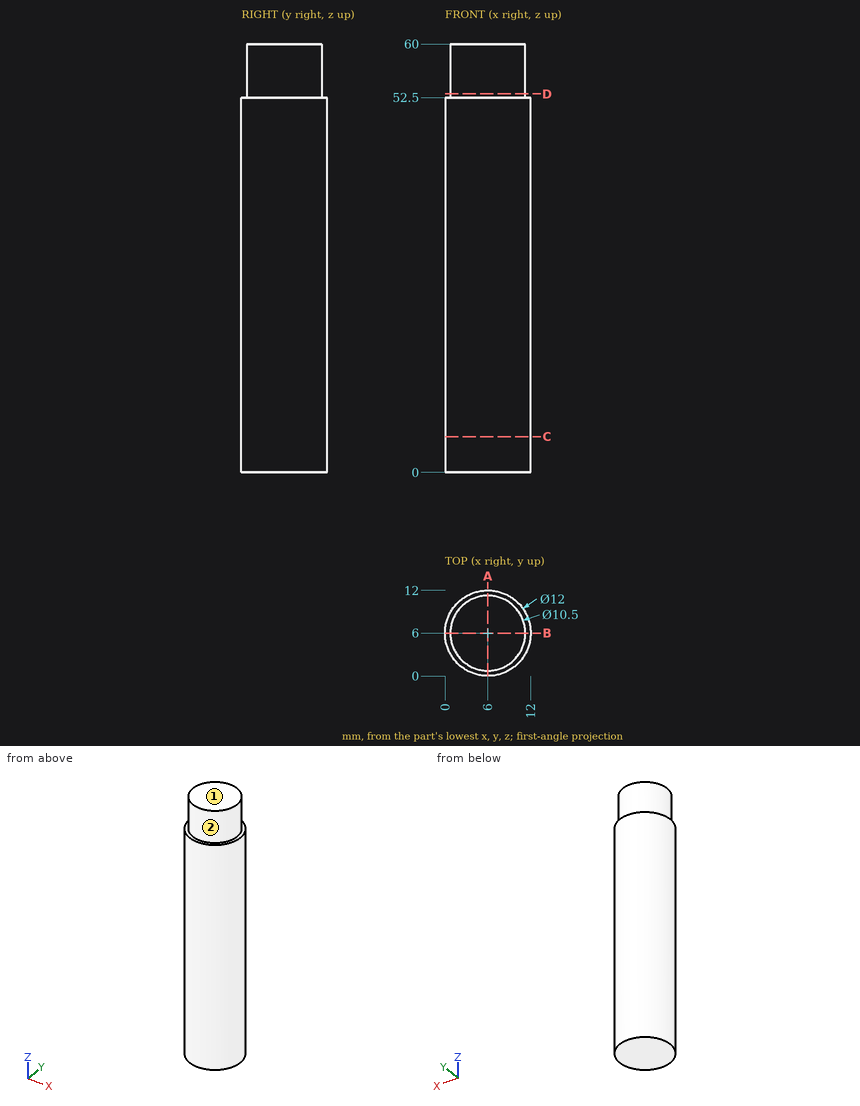
Here's the drawing with two shaded views (mm, measured from the low corner). I have some questions. A direction names the side the tool comes from. Give positions to 0.01 mm unless a question says otherwise; leave off trailing zeros. Loops run counter-clockwise (first coordinate to the right, second up) from the corner with the lowest first, then second, coordinate; pieces in that order, holes last. Notation, with made-up numbers: M 21,-31 L 72,-31 A35 cw 72,7 Z; hole C 78.25,89 d3. An arc over 180 degrees is marked long. Use one line per item in the form item = value. Start each with the question number.
(1) Please list where these lines run through material, in increasing order: line 1 (Z direction, x = 6.25, y = 11.5); line 2 (X direction, y = 5.5, z = 27); line 3 (Y direction, x = 8.75, z = 43.5).
(2) I want a section at C-C, the plane z = 5. Write out the boundary of the cut face in (x, y).
(3) I'm going to push flat-ended pins straight in: P1, Ø1, axis at x = 5, z = 40.5, coming from the -Y side; P2, Ø6, axis at y = 6, z = 53, coming from the +X side. Where does each tip first touch, or does it pass through?
(4) I want a section at D-D, the plane z = 53. Write out the boundary of the cut face in (x, y), and give its area (3 significant figures).
(5) On a 3-axis mill with a long thin cutter (end or side, diameter ignored), from which of +Z, -Z, +X, -X, +Y, -Y can I reach the whole of each face in a straight line? I mean the marked faces 1 and 2. Say none if no direction works.
(6) I want a section at A-A, the plane x = 6. Write out the boundary of the cut face in (y, z), and give its area (3 significant figures).
Worked out:
q1.line_1 = 0 to 52.5
q1.line_2 = 0.02 to 11.98
q1.line_3 = 0.67 to 11.33
q2.outline = C 6,6 d12
q3.P1 = 0.02
q3.P2 = 12
q4.outline = C 6,6 d10.5
q4.area = 86.6 mm²
q5.face_1 = +Z, +X, -X, +Y, -Y
q5.face_2 = +Z
q6.outline = M 0,0 L 12,0 L 12,52.5 L 11.25,52.5 L 11.25,60 L 0.75,60 L 0.75,52.5 L 0,52.5 Z
q6.area = 709 mm²
